```python
from build123d import *

# Parameters (mm, degrees)
SKETCH1_R           = 15.875
BOSS_EXTRUDE1_DEPTH = 88.9
BOSS_EXTRUDE2_DEPTH = 4
SKETCH3_R           = 9.999999939
BOSS_EXTRUDE3_DEPTH = 27.99999991


with BuildPart() as part:
    # Sketch1 → Boss-Extrude1 (new body)
    with BuildSketch(Plane(origin=(0, 0, 0), x_dir=(1, 0, 0), z_dir=(0, 1, 0))):
        Circle(SKETCH1_R)
    extrude(amount=BOSS_EXTRUDE1_DEPTH)

    # Sketch2 → Boss-Extrude2 (add)
    with BuildSketch(Plane(origin=(0, 88.9, 0), x_dir=(1, 0, 0), z_dir=(0, 1, 0))):
        with BuildLine():
            Line((-18.875, 0), (-18.875, 20.32))
            ThreePointArc((-18.875, 20.32), (0, 39.195), (18.875, 20.32))
            Line((18.875, 20.32), (18.875, 0))
            ThreePointArc((18.875, 0), (0, -18.875), (-18.875, 0))
        make_face()
    extrude(amount=BOSS_EXTRUDE2_DEPTH)

    # Sketch3 → Boss-Extrude3 (add)
    with BuildSketch(Plane.XZ):
        Circle(SKETCH3_R)
    extrude(amount=BOSS_EXTRUDE3_DEPTH)


solid = part.part
```
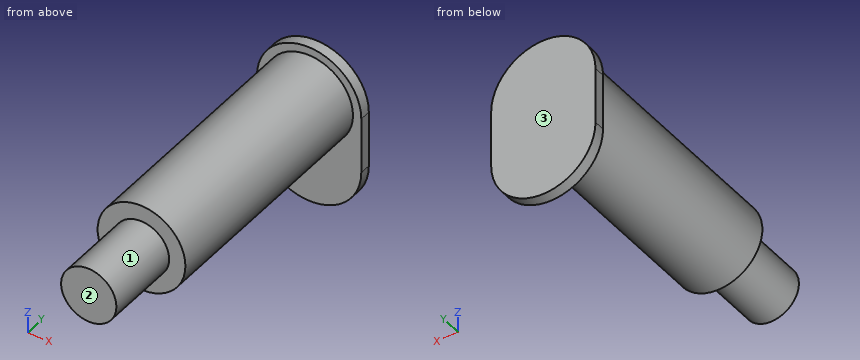
Check sheet for the modelled part. Datum: model origin and axes. Units: mm. Face numbers are marked on the shaded views. Coordinates: 2 decimals unless noted, no trailing zeros. Write each loop counter-clockwise with the first axis right and the second up, starting at its lowest first coordinate (ties: lowest second). Pieces come first, ordered by that corner, then holes. Notation, with made-up numbers: M 39,-20.75 L 85,-20.75 A32 cw 85,18.25 Z; hole C -5.75,-11 d1. An arc over 180 degrees is marked long. Use one line per item in the form item = value.
Item 1: Sectioned sample at B-B, the plane z = -7. Record the cut outline in (x, y) (3 decimals), and give its area (3 significant figures).
Answer below:
outline = M -18.875,88.9 L -14.248,88.9 L -14.248,0 L -7.141,0 L -7.141,-28 L 7.141,-28 L 7.141,0 L 14.248,0 L 14.248,88.9 L 18.875,88.9 L 18.875,92.9 L -18.875,92.9 Z
area = 3,080 mm^2
Item 2: Gauge pin test, flat ends, axial feed: pin 1 Ø1 at (x, y) = (9, -12.5) entering from -Z; pin 2 Ø5 at (x, y) = (-6.5, 16) entering from -Z; pin 3 Ø12 at (x, y) = (-10, 28) entering from +Z. Record the tip position at first contact, or that the pin passes through.
Answer below:
pin_1 = -5.27
pin_2 = -15.36
pin_3 = 15.36
Item 3: Sectioned sample at D-D, the plane x = 14. Record the cut outline in (y, z).
Answer below:
outline = M 0,-7.48 L 88.9,-7.48 L 88.9,-32.98 L 92.9,-32.98 L 92.9,12.66 L 88.9,12.66 L 88.9,7.48 L 0,7.48 Z
Item 4: Sectioned sample at A-A, the plane x = 0. Record the cut outline in (y, z) (3 decimals), and give its area (3 significant figures).
Answer below:
outline = M -28,-10 L 0,-10 L 0,-15.875 L 88.9,-15.875 L 88.9,-39.195 L 92.9,-39.195 L 92.9,18.875 L 88.9,18.875 L 88.9,15.875 L 0,15.875 L 0,10 L -28,10 Z
area = 3,610 mm^2
Item 5: Sectioned sample at C-C, the plane y = 68. Record the cut outline in (x, z) (3 decimals).
Answer below:
outline = C 0,0 d31.75
Item 6: Release check for a two-part mould opening along Y. For the marked faces 1, 2 and 3 record: pulls with the +Y half, pulls with the -Y half, needs draft (parallel to the pull), parting line crosses it, or undercut.
Answer below:
face_1 = needs draft
face_2 = pulls with the -Y half
face_3 = pulls with the +Y half
Item 7: Material ranges on L1, parallel to Z at x = -0.5, y = 7; L2, parallel to Y at x = 9.5, z = -34; L3, parallel to Y at x = -5.5, z = 9, recorded low to high. Write a range as from..to.
Answer below:
L1 = -15.87..15.87
L2 = 88.9..92.9
L3 = 0..92.9
